Autodesk Inventor part; units mm, degrees
ref_plane "YZ Plane" through (0, 0, 0) normal (1, 0, 0) x (0, 1, 0)
ref_plane "XZ Plane" through (0, 0, 0) normal (0, 1, 0) x (-1, 0, 0)
ref_plane "XY Plane" through (0, 0, 0) normal (0, 0, 1) x (1, 0, 0)
sketch "Sketch1" plane through (0, 0, 0) normal (0, 0, 1) x (1, 0, 0)
  line L0 (113.6513, 30) -> (113.6513, 12)
  line L1 (113.6513, 12) -> (99.9513, 12)
  line L2 (99.9513, 12) -> (99.9513, 30)
  line L3 (99.9513, 30) -> (99.8013, 30)
  line L4 (99.8013, -3.4599) -> (99.8013, 30)
  line L5 (113.8013, -3.4599) -> (99.8013, -3.4599)
  line L6 (113.8013, 30) -> (113.8013, -3.4599)
  line L7 (113.8013, 30) -> (113.6513, 30)
  line L8 (96.8013, 30) -> (96.8013, -2.4219)
  line L9 (116.8013, 30) -> (116.8013, -2.4219)
  line L10 (116.8013, -2.4219) -> (96.8013, -2.4219)
  line L11 (96.8013, 30) -> (99.8013, 30)
  line L12 (113.8013, 30) -> (116.8013, 30)
  point P0 (0, 0)
  point P1 (99.8013, -2.4219)
  point P2 (113.8013, -2.4219)
extrude "Extrusion1" add sketch "Sketch1" along normal blind 2 contours L7 L6 L10 L4 L3 L2 L1 L0 | L12 L9 L10 L6 | L10 L8 L11 L4
equation "\"BendRadius\" = Thickness"
equation "\"BendReliefWidth\" = Thickness"
equation "\"BendReliefDepth\" = 0.5 * Thickness"
equation "\"CornerReliefSize\" = 4 * Thickness"
equation "\"MinimumRemnant\" = 2 * Thickness"
equation "\"TransitionRadius\" = BendRadius"
equation "\"JacobiRadiusSize\" = BendRadius"
equation "\"GapSize\" = Thickness"
properties part number "BackWheelMotorMountSpacer" material "Steel, Mild"
Can you work these out from the model? Positions are in its coordinate system, mm. A direction names the side the tool comes from. Give positions to 0.01 mm unless a question says otherwise; leave off trailing zeros. Loops run counter-clockwise (first coordinate to the right, second up) from the corner with the lowest first, then second, coordinate; pieces in that order, holes last. Notation, with made-up numbers: (57, 52.25) - (66, 52.25) arc R14 ccw to (66, 78.25) - close; hole circle Ø5 at (-5, 35). An arc over 180 degrees is marked (long way). One line per item, written item: value.
(1) I need wall thicknesses on line 1 along X through (y, z) = (18, 0.9); line 2 along Y through (x, z) = (101.25, 1.2). Which ranges of each line are inside material? Lowest first, please.
Verdict:
line 1: 96.8 to 99.95, 113.65 to 116.8
line 2: -2.42 to 12
(2) If we section it at C-C, the plane x = 103.5: List the corners of the cut face in (y, z) for me, plus the area to 3 significant figures.
Verdict:
outline: (-2.42, 0) - (12, 0) - (12, 2) - (-2.42, 2) - close
area: 28.8 mm^2
(3) If we section it at A-A, the plane z = 0.4: List the corners of the cut face in (x, y) for me, plus the area to 3 significant figures.
Verdict:
outline: (96.8, -2.42) - (116.8, -2.42) - (116.8, 30) - (113.65, 30) - (113.65, 12) - (99.95, 12) - (99.95, 30) - (96.8, 30) - close
area: 402 mm^2
(4) On a 3-axis mill with a long thin cutter (end or side, diameter ignored), from which of +Z, -Z, +X, -X, +Y, -Y can I reach the whole of each face in a straight line? I mean faces 1 (the face through (107, -2.422, 1)), 2 (the face through (113.651, 21, 1)). Say none if no direction works.
Verdict:
face 1: +Z, -Z, +X, -X, -Y
face 2: +Z, -Z, +Y
(5) If we mould it in two halves opening along X, with no side actions, what happens to faces 3 (the face through (99.951, 21, 1)), 4 (the face through (116.801, 14, 1)), 5 (the face through (107, 12, 1)), 6 (the face through (98, 30, 1))? For each: released by +X, released by -X, zero draft, split by the parting line, or undercut.
Verdict:
face 3: undercut
face 4: released by +X
face 5: undercut
face 6: zero draft
(6) I'm going to push a flat-ended pin straight in: pin 1 (1 mm diameter, centred on x = 108, z = 1, fed in from +Y). Where does the tip first touch, or does it pass through?
Verdict:
pin 1: y = 12
(7) If we section it at B-B, the plane y = 23: List the corners of the cut face in (x, z) for me.
Verdict:
outline: (96.8, 0) - (99.95, 0) - (99.95, 2) - (96.8, 2) - close; (113.65, 0) - (116.8, 0) - (116.8, 2) - (113.65, 2) - close
